```python
from build123d import *

# Parameters (mm, degrees)
F0_R     = 24.9326348986
F1_DEPTH = 40.2336
F2_R     = 10.16
F3_DEPTH = 15.7734
F4_R     = 3.302


with BuildPart() as f1:
    # F0 (on Top) → F1 (new body)
    with BuildSketch(Plane.XY):
        with BuildLine():
            ThreePointArc((9.5121844836, -26.9452959039), (23.3274655355, -16.5033322905), (28.575, 0))
            ThreePointArc((28.575, 0), (23.3274655355, 16.5033322905), (9.5121844836, 26.9452959039))
            ThreePointArc((9.5121844836, 26.9452959039), (-28.575, 0), (9.5121844836, -26.9452959039))
        make_face()
        Circle(F0_R, mode=Mode.SUBTRACT)
        Circle(F0_R)
        with BuildLine():
            ThreePointArc((14.2048280027, -4.8514), (-15.0104370538, 0), (14.2048280027, 4.8514))
            Line((14.2048280027, 4.8514), (17.8063629462, 4.8514))
            Line((17.8063629462, 4.8514), (17.8063629462, -4.8514))
            Line((17.8063629462, -4.8514), (14.2048280027, -4.8514))
        make_face(mode=Mode.SUBTRACT)
    extrude(amount=F1_DEPTH)

    # F2 (on face) → F3 (join)
    with BuildSketch(Plane.XY):
        with BuildLine():
            Line((57.1919272622, 18.7764181619), (9.5121844836, 26.9452959039))
            ThreePointArc((9.5121844836, 26.9452959039), (23.3274655355, 16.5033322905), (28.575, 0))
            ThreePointArc((28.575, 0), (23.3274655355, -16.5033322905), (9.5121844836, -26.9452959039))
            Line((9.5121844836, -26.9452959039), (57.1919272622, -18.7764181619))
            ThreePointArc((57.1919272622, -18.7764181619), (73.025, 0), (57.1919272622, 18.7764181619))
        make_face()
        with Locations((53.975, 0)):
            Circle(F2_R, mode=Mode.SUBTRACT)
    extrude(amount=F3_DEPTH)

    # F4
    f4_edges = [f1.edges().sort_by_distance(p)[0] for p in [
        (-28.575, 0, 40.2336),
    ]]
    fillet(f4_edges, radius=F4_R)


solid = f1.part
```
Input: part model. Units: mm. Frame: model coordinates. A direction names the side the tool comes from. Coordinates: 2 decimals unless noted, no trailing zeros. Order: outer loops, then holes, each group sorted by start corner. A loop starts at its lowest first (then second) coordinate and runs counter-clockwise, first axis right, second up. Notation, with made-up numbers: (-7, 21) - (44, 21) arc R18 cw to (44, 47) - close; hole circle Ø3 at (2, 76.5). An arc over 180 degrees is marked (long way). Return JSON: item names as keys, results as strings.
Q1. First-contact query: pin 1 (4 mm diameter, centred on x = 29, y = -5, fed in from -Z); pin 2 (2 mm diameter, centred on x = -12, z = 28.5, fed in from +Y); pin 3 (1.1 mm diameter, centred on x = 15.5, z = 19.5, fed in from -Y); pin 4 (3 mm diameter, centred on x = 16, z = 14, fed in from +Y). Flat tips, straight axial feed; report the tip coordinate or a pass-through.
The answers:
{"pin 1": "stops at z = 0", "pin 2": "stops at y = 26.37", "pin 3": "stops at y = -24.35", "pin 4": "stops at y = 26.09"}
Q2. Cut plane A-A (z = 11). Return loops of the section in (x, y) (3 decimals), then the cut area to 3 significant figures.
The answers:
{"outline": "(9.512, -26.945) - (57.192, -18.776) arc R19.05 ccw to (57.192, 18.776) - (9.512, 26.945) arc R28.575 ccw (long way) to start; hole (14.205, -4.851) - (17.806, -4.851) - (17.806, 4.851) - (14.205, 4.851) arc R15.01 ccw (long way) to start; hole circle Ø20.32 at (53.975, 0)", "area": "3,380 mm2"}
Q3. Access query for faces 5 (the cylindrical face through (73.02, -0.37, 7.78)), 6 (the flat face through (17.806, 0, 20)). Directions: +Z, -Z, +X, -X, +Y, -Y. A direction counts if a zero-diameter tool reaches every point of the face in a straight line with its end or side. Return the directions, or none.
The answers:
{"face 5": "+Z, -Z, +X", "face 6": "+Z, -Z"}
Q4. Cut plane B-B (z = 20). Return loops of the section in (x, y) (3 decimals), then the cut area to 3 significant figures.
The answers:
{"outline": "circle Ø57.15 at (0, 0); hole (14.205, -4.851) - (17.806, -4.851) - (17.806, 4.851) - (14.205, 4.851) arc R15.01 ccw (long way) to start", "area": "1,830 mm2"}
Q5. Ray query, probe 1 along Y at (x, z) = (0, 9.5) (3 decimals); probe 2 along Z at (x, y) = (42.5, -18); probe 3 along Y at (x, z) = (-11, 18). Return the intervals inside material, ascending.
The answers:
{"probe 1": "y = -28.575 to -15.01, 15.01 to 28.575", "probe 2": "z = 0 to 15.77", "probe 3": "y = -26.37 to -10.21, 10.21 to 26.37"}
Q6. Cut plane C-C (x = 41). Return loops of the section in (y, z), then the cut area to 3 significant figures.
The answers:
{"outline": "(-21.55, 0) - (21.55, 0) - (21.55, 15.77) - (-21.55, 15.77) - close", "area": "680 mm2"}
Q7. Draft query along Y for faces 1 (the flat face through (22, 0, 0)), 2 (the cylindrical face through (-15, -0.6, 19.8)), 3 (the flat face through (33.018, -22.918, 7.776)), 4 (the flat face through (33.7, 22.8, 7.8)). Return one class per face: +Y half, -Y half, draft (parallel to the pull), parting line (faces both ways), or undercut.
The answers:
{"face 1": "draft", "face 2": "undercut", "face 3": "-Y half", "face 4": "+Y half"}
